from build123d import *

# Parameters (mm, degrees)
F0_W      = 170
F0_H      = 34
F1_DEPTH  = 2
F2_W      = 170
F2_H      = 2
F4_DEPTH  = 3
F5_W      = 170
F5_H      = 2
F7_DEPTH  = 3
F8_R      = 2
F9_DEPTH  = 2
F10_R     = 1
F11_DEPTH = 1
F12_R     = 3
F13_DEPTH = 1


with BuildPart() as f1:
    # F0 (on Top) → F1 (new body)
    with BuildSketch(Plane.XY):
        with Locations((-8.2408198714, -30.0435358584)):
            Rectangle(F0_W, F0_H)
    extrude(amount=F1_DEPTH)

    # F2 (on face) + F3 (on face) → F4 (join)
    with BuildSketch(Plane.XZ.offset(47.0435358584)):
        with Locations((-8.2408198714, 1)):
            Rectangle(F2_W, F2_H)
    with BuildSketch(Plane.XZ.offset(47.0435358584)):
        Polygon((75.7311444739, 0), (-92.2127468976, 0), (-8.2416068763, -163.3778810501), align=None)
    extrude(amount=F4_DEPTH)

    # F6 (on face) + F5 (on face) → F7 (join)
    with BuildSketch(Plane(origin=(0, -13.0435358584, 0), x_dir=(-1, 0, 0), z_dir=(0, 1, 0))):
        Polygon((92.2128885412, 0), (-75.7311794344, 0), (8.2415537909, -163.3778512478), align=None)
    with BuildSketch(Plane(origin=(0, -13.0435358584, 0), x_dir=(-1, 0, 0), z_dir=(0, 1, 0))):
        with Locations((8.2408198714, 1)):
            Rectangle(F5_W, F5_H)
    extrude(amount=F7_DEPTH)

    # F8 (on face) → F9 (join)
    with BuildSketch(Plane.XZ.offset(13.0435358584)):
        with Locations((-8.0062086027, -130.911280853)):
            Circle(F8_R)
    extrude(amount=F9_DEPTH)

    # F10 (on face) → F11 (cut)
    with BuildSketch(Plane.XZ.offset(15.0435358584)):
        with Locations((-8.0062086027, -130.911280853)):
            Circle(F10_R)
    extrude(amount=-F11_DEPTH, mode=Mode.SUBTRACT)

    # F12 (on face) → F13 (cut)
    with BuildSketch(Plane.XY.offset(2)):
        with Locations((-8.2408198714, -30.0435358584)):
            Circle(F12_R)
    extrude(amount=-F13_DEPTH, mode=Mode.SUBTRACT)


solid = f1.part
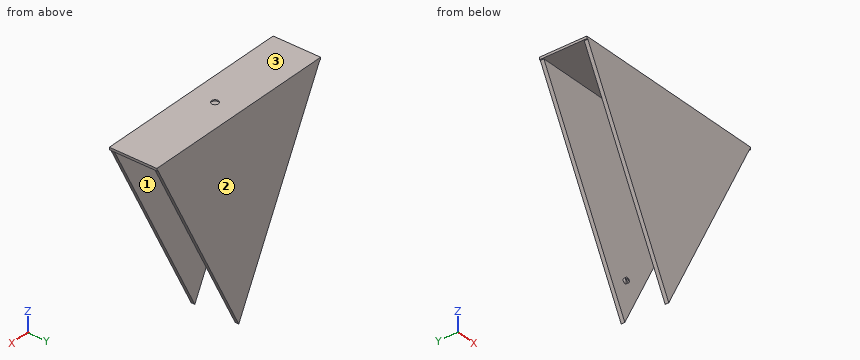
Work out the finished part from the listing and answer in its coordinate system (mm). Face numbers are marked on the shaded views. Round coordinates to 2 decimals unless told otherwise and drop trailing zeros. Write each loop counter-clockwise with the first axis right and the second up, starting at its lowest first coordinate (ties: lowest second). Pieces come first, ordered by that corner, then holes. Notation, with made-up numbers: M -21.5,3.25 L -7.5,3.25 A22 ccw -7.5,22.25 Z; hole C 48.25,2.5 d2. An arc over 180 degrees is marked long. Use a Markdown table: item, result.
1) The part is cut by section C-C on y = -44.5. Give the vertices of the cut face in (x, z), plus the area to 3 significant figures.
Taken from the geometry:
| item | result |
|---|---|
| outline | M -93.24,0 L 76.76,0 L 76.76,2 L -93.24,2 Z |
| area | 340 mm2 |
2) Flat-ended cylindrical pins translate along their axes: pin 1 (20 mm diameter, centred on x = -8.5, y = -34.5, fed in from -Z); pin 2 (1.8 mm diameter, centred on x = -7, y = -28.5, fed in from +Z). Find the tip coordinate at first contact, or state that the pin passes through.
Taken from the geometry:
| item | result |
|---|---|
| pin 1 | stops at z = 0 |
| pin 2 | stops at z = 1 |
3) The part is cut by section A-A on z = -49.5. Give the vertices of the cut face in (x, y).
Taken from the geometry:
| item | result |
|---|---|
| outline | M -66.77,-50.04 L 50.29,-50.04 L 50.29,-47.04 L -66.77,-47.04 Z; M -66.77,-13.04 L 50.29,-13.04 L 50.29,-10.04 L -66.77,-10.04 Z |
4) Determine the mould class of the marked faces 1, 2 and 3 for opening direction Y: pulls with the +Y half, pulls with the -Y half, needs draft (parallel to the pull), parting line crosses it, or undercut.
Taken from the geometry:
| item | result |
|---|---|
| face 1 | undercut |
| face 2 | pulls with the +Y half |
| face 3 | needs draft |
5) The part is cut by section B-B on x = -17. Give the vertices of the cut face in (y, z), plus the area to 3 significant figures.
Taken from the geometry:
| item | result |
|---|---|
| outline | M -50.04,-146.34 L -47.04,-146.34 L -47.04,0 L -13.04,0 L -13.04,-146.34 L -10.04,-146.34 L -10.04,2 L -50.04,2 Z |
| area | 958 mm2 |
6) The part is cut by section D-D on z = -92.5. Give the vertices of the cut face in (x, y), plus the area to 3 significant figures.
Taken from the geometry:
| item | result |
|---|---|
| outline | M -44.67,-50.04 L 28.19,-50.04 L 28.19,-47.04 L -44.67,-47.04 Z; M -44.67,-13.04 L 28.19,-13.04 L 28.19,-10.04 L -44.67,-10.04 Z |
| area | 437 mm2 |
7) Consider line 1 (Y direction, x = 18, z = -5); line 2 (Z direction, x = 63, y = -36). Determine where each line is inside the solid, lowest interval first. Write a range as [from, to].
Taken from the geometry:
| item | result |
|---|---|
| line 1 | y = [-50.04, -47.04], [-13.04, -10.04] |
| line 2 | z = [0, 2] |
